Read the model definition and answer for the solid it produces. Units are mm, in the model's axes. A direction names the side the tool comes from. Coordinates: 2 decimals unless noted, no trailing zeros. Loops run counter-clockwise (first coordinate to the right, second up) from the corner with the lowest first, then second, coordinate; pieces in that order, holes last. Notation, with made-up numbers: (2.5, 5.5) -> (12.5, 5.5) arc R25 cw to (12.5, 25.5) -> close; hole circle Ø3 at (52, 43). An arc over 180 degrees is marked (long way). Answer as a JSON object with one key per item and string values. Group by question number.
Q1. Straight lines are drawn through the part: line 1 along X through (y, z) = (48, 2); line 2 along X through (y, z) = (10, 27); line 3 along X through (y, z) = (39, 9.5). For each, find the intervals that lie inside material, in ascending order. Write a range as [from, to].
Q2. Determine the mould class of faces 1 (the flat face through (3, 60, 21)), 2 (the cylindrical face through (-44.054, 50.191, 2.535)), 3 (the cylindrical face through (36.91, 47.42, 2.54)), 4 (the flat face through (-20, 0, 14)) for opening direction Y: released by +Y, released by -Y, zero draft, split by the parting line, or undercut.
Q3. The part is cut by section D-D on y = 42.5. Write down the section's boundary in (x, z), and give its area (3 significant figures).
Q4. Each of these flat-tipped pins is pushed along its axis until it touches: P1, Ø5.5, axis at y = 13.5, z = 22.5, coming from the -X side; P2, Ø2.5, axis at x = 35, z = 1.5, coming from the -Y side; P3, Ø4, axis at y = 50.5, z = 18.5, coming from the +X side. Where does it stop, or does it pass through?
Q5. For faces 5 (the flat face through (-35, 48, 5)), 6 (the flat face through (-10, 10, 23)), 7 (the flat face through (35, 50, 5)), determine the directions among +Z, -Z, +X, -X, +Y, -Y from which every point of the face is accessible in a straight line to the end or side of a thin tool.
Q6. The part is cut by section C-C on y = 28.5. Write down the section's boundary in (x, z).
Q7. The part is cut by section A-A on y = 50. Write down the section's boundary in (x, z).
Q8. The part is cut by section B-B on z = 11.5. Write down the section's boundary in (x, y), and give its area (3 significant figures).
from build123d import *

# Parameters (mm, degrees)
F1_DEPTH = 60
F3_DEPTH = 5
F4_R     = 4.244669
F4_R_2   = 4.337045
F5_DEPTH = 5
F7_DEPTH = 30


with BuildPart() as f1:
    # F0 (on Front) → F1 (new body)
    with BuildSketch(Plane.XZ):
        with BuildLine():
            Line((20, 0), (30, 0))
            ThreePointArc((30, 0), (0, 30), (-30, 0))
            Line((-30, 0), (-20, 0))
            ThreePointArc((-20, 0), (0, 20), (20, 0))
        make_face()
    extrude(amount=-F1_DEPTH)

    # F2 (on Top) → F3 (join)
    with BuildSketch(Plane.XY):
        with BuildLine():
            Line((26, 40), (40, 40))
            ThreePointArc((40, 40), (50, 50), (40, 60))
            Line((40, 60), (26, 60))
            Line((26, 60), (26, 40))
        make_face()
        with BuildLine():
            Line((-39.86631, 60), (-39.866316, 59.999106))
            ThreePointArc((-39.866316, 59.999106), (-49.999777, 50.066844), (-40, 40))
            Line((-40, 40), (-26, 40))
            Line((-26, 40), (-26, 60))
            Line((-26, 60), (-39.86631, 60))
        make_face()
    extrude(amount=F3_DEPTH)

    # F4 (on face) → F5 (cut)
    with BuildSketch(Plane.XY.offset(5)):
        with Locations((40.278634, 50)):
            Circle(F4_R)
        with Locations((-39.721366, 50)):
            Circle(F4_R_2)
    extrude(amount=-F5_DEPTH, mode=Mode.SUBTRACT)

    # F6 (on Top) → F7 (cut)
    with BuildSketch(Plane.XY):
        with BuildLine():
            Line((10, 0), (10, 20))
            ThreePointArc((10, 20), (0, 30), (-10, 20))
            Line((-10, 20), (-10, 0))
            Line((-10, 0), (10, 0))
        make_face()
    extrude(amount=F7_DEPTH, mode=Mode.SUBTRACT)


solid = f1.part
Final values:
{
 "1": {"line 1": "x = [-49.8, -43.57], [-35.87, -19.9], [19.9, 36.53], [44.02, 49.8]", "line 2": "x = [-13.08, -10], [10, 13.08]", "line 3": "x = [-28.46, -17.6], [17.6, 28.46]"},
 "2": {"face 1": "released by +Y", "face 2": "undercut", "face 3": "undercut", "face 4": "released by -Y"},
 "3": {"outline": "(-46.61, 0) -> (-20, 0) arc R20 cw to (20, 0) -> (46.61, 0) -> (46.61, 5) -> (29.58, 5) arc R30 ccw to (-29.58, 5) -> (-46.61, 5) -> close", "area": "953 mm2"},
 "4": {"P1": "stops at x = -22.58", "P2": "stops at y = 40", "P3": "stops at x = 25.05"},
 "5": {"face 5": "+Z, -X, +Y, -Y", "face 6": "+Z, -Z, -Y", "face 7": "+Z, +X, +Y, -Y"},
 "6": {"outline": "(-30, 0) -> (-20, 0) arc R20 cw to (-5.27, 19.29) -> (-5.27, 29.53) arc R30 ccw to start; (5.27, 19.29) arc R20 cw to (20, 0) -> (30, 0) arc R30 ccw to (5.27, 29.53) -> close"},
 "7": {"outline": "(-50, 0) -> (-44.06, 0) -> (-44.06, 5) -> (-50, 5) -> close; (-35.38, 0) -> (-20, 0) arc R20 cw to (20, 0) -> (36.03, 0) -> (36.03, 5) -> (29.58, 5) arc R30 ccw to (-29.58, 5) -> (-35.38, 5) -> close; (44.52, 0) -> (50, 0) -> (50, 5) -> (44.52, 5) -> close"},
 "8": {"outline": "(-27.71, 0) -> (-16.36, 0) -> (-16.36, 60) -> (-27.71, 60) -> close; (16.36, 0) -> (27.71, 0) -> (27.71, 60) -> (16.36, 60) -> close", "area": "1,360 mm2"}
}
